Could you check a few things on this model? Use its own coordinates, in mm. Face numbers are marked on the shaded views. A direction names the side the tool comes from. Coordinates: 2 decimals unless noted, no trailing zeros. Write each loop counter-clockwise with the first axis right and the second up, starting at its lowest first coordinate (ties: lowest second). Pieces come first, ordered by that corner, then holes.
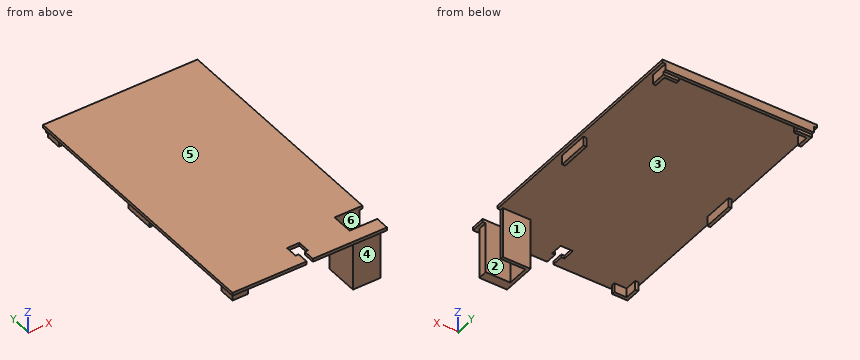
```python
from build123d import *

# Parameters (mm, degrees)
SKETCH1_W           = 100
SKETCH1_H           = 177.5
BOSS_EXTRUDE1_DEPTH = 2
SKETCH3_W           = 2
SKETCH3_H           = 20
BOSS_EXTRUDE2_DEPTH = 6
SKETCH4_W           = 96
SKETCH4_H           = 2
BOSS_EXTRUDE3_DEPTH = 4
BOSS_EXTRUDE5_DEPTH = 33
SKETCH7_W           = 18
SKETCH7_H           = 14
CUT_EXTRUDE2_DEPTH  = 207.386167172
CUT_EXTRUDE3_DEPTH  = 207.386167172


with BuildPart() as part:
    # Sketch1 → Boss-Extrude1 (new body)
    with BuildSketch(Plane.XY):
        with Locations((50, 88.75)):
            Rectangle(SKETCH1_W, SKETCH1_H)
    extrude(amount=BOSS_EXTRUDE1_DEPTH)

    # Sketch3 → Boss-Extrude2 (add)
    with BuildSketch(Plane(origin=(0, 0, 0), x_dir=(-1, 0, 0), z_dir=(0, 0, -1))):
        Polygon((-98, 175.5), (-88, 175.5), (-88, 173.5), (-96, 173.5), (-96, 165.5), (-98, 165.5), align=None)
        Polygon((-12, 175.5), (-2, 175.5), (-2, 165.5), (-4, 165.5), (-4, 173.5), (-12, 173.5), align=None)
        Polygon((-2, 3), (-12, 3), (-12, 5), (-4, 5), (-4, 13), (-2, 13), align=None)
        with Locations((-97, 90.5)):
            Rectangle(SKETCH3_W, SKETCH3_H)
        with Locations((-3, 90.5)):
            Rectangle(SKETCH3_W, SKETCH3_H)
    extrude(amount=BOSS_EXTRUDE2_DEPTH)

    # Sketch4 → Boss-Extrude3 (add)
    with BuildSketch(Plane(origin=(0, 0, 0), x_dir=(-1, 0, 0), z_dir=(0, 0, -1))):
        with Locations((-50, 176.5)):
            Rectangle(SKETCH4_W, SKETCH4_H)
    extrude(amount=BOSS_EXTRUDE3_DEPTH)

    # Sketch5 → Boss-Extrude5 (add)
    with BuildSketch(Plane(origin=(0, 0, 0), x_dir=(-1, 0, 0), z_dir=(0, 0, -1))):
        Polygon((-98, 3), (-80, 3), (-80, 25), (-98, 25), (-98, 23), (-82, 23), (-82, 9), (-98, 9), align=None)
    extrude(amount=BOSS_EXTRUDE5_DEPTH)

    # Sketch7 → Cut-Extrude2 (cut, through all)
    with BuildSketch(Plane(origin=(0, 0, 0), x_dir=(-1, 0, 0), z_dir=(0, 0, -1))):
        with Locations((-91, 16)):
            Rectangle(SKETCH7_W, SKETCH7_H)
    extrude(amount=-CUT_EXTRUDE2_DEPTH, mode=Mode.SUBTRACT)

    # Sketch8 → Cut-Extrude3 (cut, through all)
    with BuildSketch(Plane(origin=(0, 0, 0), x_dir=(-1, 0, 0), z_dir=(0, 0, -1))):
        Polygon((-48, 0), (-48, 7.5), (-46, 7.5), (-46, 15.5), (-54, 15.5), (-54, 7.5), (-52, 7.5), (-52, 0), align=None)
    extrude(amount=-CUT_EXTRUDE3_DEPTH, mode=Mode.SUBTRACT)


solid = part.part
```
1. I want a section at B-B on z = -25.5. Please give me the cut outline in (x, y), plus the area to 3 significant figures.
Verdict:
outline: (80, 3) - (98, 3) - (98, 9) - (82, 9) - (82, 23) - (98, 23) - (98, 25) - (80, 25) - close
area: 172 mm2
2. Please list where these lines run through material, in increasing order: line 1 along Y through (x, z) = (89.5, -12); line 2 along X through (y, z) = (166.5, -4.5); line 3 along Z through (x, y) = (81, 82).
Verdict:
line 1: y = 3 to 9, 23 to 25
line 2: x = 2 to 4, 96 to 98
line 3: z = 0 to 2
3. If we mould it in two halves opening along Y, with no side actions, what happens to the marked faces 3, 4, 5 and 6? For each: pulls with the +Y half, pulls with the -Y half, needs draft (parallel to the pull), parting line crosses it, or undercut.
Verdict:
face 3: undercut
face 4: pulls with the -Y half
face 5: needs draft
face 6: undercut
4. I want a section at A-A on x = 92. Please give me the cut outline in (y, z).
Verdict:
outline: (0, 0) - (3, 0) - (3, -33) - (9, -33) - (9, 2) - (0, 2) - close; (23, -33) - (25, -33) - (25, 0) - (173.5, 0) - (173.5, -6) - (175.5, -6) - (175.5, -4) - (177.5, -4) - (177.5, 2) - (23, 2) - close
5. On a 3-axis mill with a long thin cutter (end or side, diameter ignored), from which of +Z, -Z, +X, -X, +Y, -Y can I reach the whole of each face in a straight line? I mean the marked faces 1 and 2. Say none if no direction works.
Verdict:
face 1: -Z, +X, -X
face 2: +Z, -Z, +X
6. I want a section at D-D on x = 77. Please give me the cut outline in (y, z).
Verdict:
outline: (0, 0) - (175.5, 0) - (175.5, -4) - (177.5, -4) - (177.5, 2) - (0, 2) - close
7. For pin 1 (1 mm diameter, centred on y = 11, z = 1.5, fed in from -X); pin 2 (6.5 mm diameter, centred on y = 170.5, z = -3.5, fed in from +X); pin 3 (1.6 mm diameter, centred on x = 97.5, z = -1.5, fed in from -Y); pin 4 (5 mm diameter, centred on x = 68.5, y = 119, fed in from -Z), each with a flat end and sliding along its axis, tell me the tip position at first contact or that it passes through.
Verdict:
pin 1: stops at x = 0
pin 2: stops at x = 98
pin 3: stops at y = 3
pin 4: stops at z = 0
8. I want a section at C-C on y = 97.5. Please give me the cut outline in (x, z).
Verdict:
outline: (0, 0) - (2, 0) - (2, -6) - (4, -6) - (4, 0) - (96, 0) - (96, -6) - (98, -6) - (98, 0) - (100, 0) - (100, 2) - (0, 2) - close
